from build123d import *

# Parameters (mm, degrees)
F0_W     = 12.7
F0_H     = 20.32
F1_DEPTH = 5.08
F2_W     = 12.7
F2_H     = 4.4710185971
F3_DEPTH = 6.35
F5_DEPTH = 25.4
F6_W     = 16.4084
F6_H     = 3.556
F7_DEPTH = 25.4


with BuildPart() as f1:
    # F0 (on Top) → F1 (new body)
    with BuildSketch(Plane.XY):
        with Locations((0, 2.5246988346)):
            Rectangle(F0_W, F0_H)
    extrude(amount=F1_DEPTH)

    # F2 (on face) → F3 (join)
    with BuildSketch(Plane.XY.offset(5.08)):
        with Locations((0, 10.4491895361)):
            Rectangle(F2_W, F2_H)
    extrude(amount=F3_DEPTH)

    # F4 (on face) → F5 (cut)
    with BuildSketch(Plane.YZ.offset(6.35)):
        with BuildLine():
            ThreePointArc((8.2136802375, 5.08), (8.788877567, 8.4460066037), (10.4491895361, 11.43))
            Line((10.4491895361, 11.43), (8.2136802375, 11.43))
            Line((8.2136802375, 11.43), (8.2136802375, 5.08))
        make_face()
    extrude(amount=-F5_DEPTH, mode=Mode.SUBTRACT)

    # F6 (on face) → F7 (cut)
    with BuildSketch(Plane.YZ.offset(6.35)):
        with Locations((2.5246988346, 1.778)):
            Rectangle(F6_W, F6_H)
    extrude(amount=-F7_DEPTH, mode=Mode.SUBTRACT)


solid = f1.part
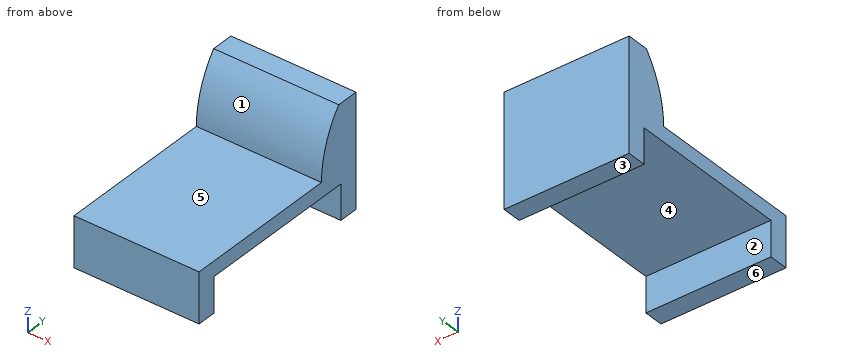
Geometry: final body of the model. Coordinates: model frame, mm. Face numbers are marked on the shaded views. A direction names the side the tool comes from. Round coordinates to 2 decimals unless told otherwise and drop trailing zeros. Order: outer loops, then holes, each group sorted by start corner. A loop starts at its lowest first (then second) coordinate and runs counter-clockwise, first axis right, second up. Notation, with made-up numbers: (88, 18.25) - (135, 18.25) arc R21 ccw to (135, 41.25) - close; hole circle Ø1 at (41, 35.25). An arc over 180 degrees is marked (long way). Write each question's results on one line, items separated by ' | '.
Item 1: Section A-A, the plane z = 2.5. Return the cut outline in (x, y), and give its area (3 significant figures).
Completed:
outline: (-6.35, -7.64) - (6.35, -7.64) - (6.35, -5.68) - (-6.35, -5.68) - close; (-6.35, 10.73) - (6.35, 10.73) - (6.35, 12.68) - (-6.35, 12.68) - close | area: 49.7 mm^2
Item 2: Reachability of the marked faces 4, 5 and 6 from +Z, -Z, +X, -X, +Y, -Y: full face, straight path, thin tool, end or side. Return the list, or none.
Completed:
face 4: -Z, +X, -X | face 5: +Z, +X, -X, -Y | face 6: -Z, +X, -X, +Y, -Y
Item 3: First-contact query: pin 1 Ø4 at (x, y) = (-0.5, 4) entering from +Z; pin 2 Ø1.5 at (x, y) = (-2.5, 9.5) entering from +Z; pin 3 Ø2 at (x, z) = (-4.5, 7) entering from -Y. Flat tips, straight axial feed; report the tip coordinate or a pass-through.
Completed:
pin 1: z = 5.08 | pin 2: z = 11.17 | pin 3: y = 8.26
Item 4: Section D-D, the plane z = 6. Return the cut outline in (x, y).
Completed:
outline: (-6.35, 8.26) - (6.35, 8.26) - (6.35, 12.68) - (-6.35, 12.68) - close
Item 5: Material intervals for line 1 along Y through (x, z) = (2.75, 2); line 2 along Z through (x, y) = (-5.5, 0.25); line 3 along Y through (x, z) = (0, 6), sorted ascending. Write a range as [from, to].
Completed:
line 1: [-7.64, -5.68], [10.73, 12.68] | line 2: [3.56, 5.08] | line 3: [8.26, 12.68]
Item 6: Section B-B, the plane x = -2.75. Return the cut outline in (y, z), and give its area (3 significant figures).
Completed:
outline: (-7.64, 0) - (-5.68, 0) - (-5.68, 3.56) - (10.73, 3.56) - (10.73, 0) - (12.68, 0) - (12.68, 11.43) - (10.45, 11.43) arc R10.14 ccw to (8.21, 5.08) - (-7.64, 5.08) - close | area: 68.8 mm^2
Item 7: Section C-C, the plane y = -6.5. Return the cut outline in (x, z).
Completed:
outline: (-6.35, 0) - (6.35, 0) - (6.35, 5.08) - (-6.35, 5.08) - close
Item 8: Mould query, pull axis Y, two halves, no side actions, for the marked faces 1, 2 and 3. Classes: pulls with the +Y half, pulls with the -Y half, needs draft (parallel to the pull), parting line crosses it, or undercut.
Completed:
face 1: pulls with the -Y half | face 2: undercut | face 3: needs draft
